Read the model definition and answer for the solid it produces. Units are mm, in the model's axes. Coordinates: 2 decimals unless noted, no trailing zeros. Write each loop counter-clockwise with the first axis right and the second up, starting at its lowest first coordinate (ties: lowest second). Pieces come first, ordered by that corner, then holes. Notation, with made-up numbers: (58.5, 52.5) -> (103.5, 52.5) arc R19 ccw to (103.5, 68.5) -> close; hole circle Ø1 at (-24.5, 12.5). An arc over 180 degrees is marked (long way). One line per item, written item: value. Start each with the question number.
1. Find section B-B, the plane x = 82. Write down the section's boundary in (y, z).
2. Consider line 1 along X through (y, z) = (1.3, -12); line 2 along Z through (x, y) = (11, 0.9); line 3 along X through (y, z) = (1.5, -50.5) (3 decimals). Determine where each line is inside the solid, lowest interval first.
3. Given P1, Ø3.5, axis at x = 82, z = -44, coming from the -Y side, flat-ended and moving along its own axis, determine where the tip first touches the part or whether it passes through.
4. Find section C-C, the plane y = 3.9. State how many separate pieces and enclosed holes the cut face has, and give its area (3 significant figures).
5. Find section A-A, the plane z = -12. Write down the section's boundary in (x, y), and give its area (3 significant figures).
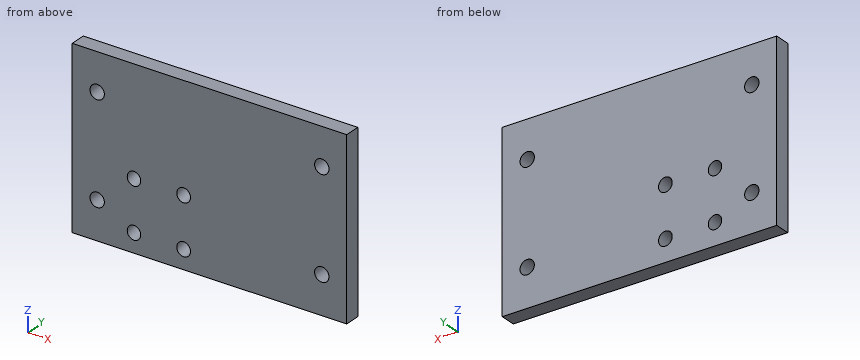
```python
from build123d import *

# Parameters (mm, degrees)
SKETCH1_W           = 90
SKETCH1_H           = 56.23
BOSS_EXTRUDE1_DEPTH = 5
SKETCH2_R           = 2.3
CUT_EXTRUDE1_DEPTH  = 15
SKETCH7_R           = 2.3
CUT_EXTRUDE3_DEPTH  = 45
SKETCH9_W           = 61.183864123
SKETCH9_H           = 5.04390519
CUT_EXTRUDE4_DEPTH  = 2
SKETCH11_R          = 2.159579804
SKETCH11_R_2        = 2.2
SKETCH11_R_3        = 2.200145532
CUT_EXTRUDE5_DEPTH  = 20


with BuildPart() as part:
    # Sketch1 → Boss-Extrude1 (new body)
    with BuildSketch(Plane(origin=(0, 0, 0), x_dir=(1, 0, 0), z_dir=(0, 1, 0))):
        with Locations((45, 28.115)):
            Rectangle(SKETCH1_W, SKETCH1_H)
    extrude(amount=BOSS_EXTRUDE1_DEPTH)

    # Sketch2 → Cut-Extrude1 (cut)
    with BuildSketch(Plane(origin=(0, 5, 0), x_dir=(1, 0, 0), z_dir=(0, 1, 0))):
        with Locations(Location((82, 12, 0), (0, 0, 270))):
            Circle(SKETCH2_R)
        with Locations(Location((10, 12, 0), (0, 0, 270))):
            Circle(SKETCH2_R)
    extrude(amount=-CUT_EXTRUDE1_DEPTH, mode=Mode.SUBTRACT)

    # Sketch7 → Cut-Extrude3 (cut)
    with BuildSketch(Plane(origin=(0, 5, 0), x_dir=(1, 0, 0), z_dir=(0, 1, 0))):
        with Locations(Location((82, 44, 0), (0, 0, 270))):
            Circle(SKETCH7_R)
        with Locations(Location((10, 44, 0), (0, 0, 270))):
            Circle(SKETCH7_R)
    extrude(amount=-CUT_EXTRUDE3_DEPTH, mode=Mode.SUBTRACT)

    # Sketch9 → Cut-Extrude4 (cut)
    with BuildSketch(Plane.ZY):
        with Locations((-25.638067939, 2.521952595)):
            Rectangle(SKETCH9_W, SKETCH9_H)
    extrude(amount=-CUT_EXTRUDE4_DEPTH, mode=Mode.SUBTRACT)

    # Sketch11 → Cut-Extrude5 (cut)
    with BuildSketch(Plane(origin=(0, 4.817959636, 0.936516484), x_dir=(1, 0, 0), z_dir=(0, 0.9816271834476639, 0.19080899537654525))):
        with Locations(Location((21.790317182, 49.227295285, 0), (0, 0, 270))):
            Circle(SKETCH11_R)
        with Locations(Location((37.700491288, 49.227295285, 0), (0, 0, 270))):
            Circle(SKETCH11_R_2)
        with Locations(Location((37.700491288, 33.498951741, 0), (0, 0, 270))):
            Circle(SKETCH11_R_3)
        with Locations(Location((21.790317182, 33.498951741, 0), (0, 0, 270))):
            Circle(SKETCH11_R)
    extrude(amount=-CUT_EXTRUDE5_DEPTH, mode=Mode.SUBTRACT)


solid = part.part
```
Answer block:
1. outline: (0, -56.23) -> (5, -56.23) -> (5, -46.3) -> (0, -46.3) -> close; (0, -41.7) -> (5, -41.7) -> (5, -14.3) -> (0, -14.3) -> close; (0, -9.7) -> (5, -9.7) -> (5, 0) -> (0, 0) -> close
2. line 1: x = 2 to 7.7, 12.3 to 79.7, 84.3 to 90
2. line 2: z = -56.23 to -46.07, -41.93 to -14.07, -9.93 to 0
2. line 3: x = 2 to 19.725, 23.856 to 35.593, 39.808 to 90
3. P1: passes through
4. separate pieces: 1
4. enclosed holes: 8
4. area: 4,820 mm2
5. outline: (2, 0) -> (7.7, 0) -> (7.7, 5) -> (2, 5) -> close; (12.3, 0) -> (79.7, 0) -> (79.7, 5) -> (12.3, 5) -> close; (84.3, 0) -> (90, 0) -> (90, 5) -> (84.3, 5) -> close
5. area: 394 mm2
